Input: dimensioned drawing with shaded views. Units: mm. Origin: part minimum x, y, z. A direction names the side the tool comes from. Round coordinates to 2 decimals unless told otherwise and drop trailing zeros. Loops run counter-clockwise (first coordinate to the right, second up) from the corner with the lowest first, then second, coordinate; pieces in that order, holes last. Notation, with made-up numbers: M -7.75,-24.5 L 19.25,-24.5 A16 ccw 19.25,-15.5 Z; hole C 35,54.5 d7. An arc over 180 degrees is marked long. Write each question's results on one line, items separated by ' | '. Start each with the question number.
1. Section D-D on x = 3. Output: boundary loops of the cut face in (y, z).
2. Draft query along X for the marked faces 1, 2 and 3. Return one class per face: released by +X, released by -X, zero draft, split by the parting line, or undercut.
3. Set-up query: the marked faces 4, 5 and 6. Return all of +Z, -Z, +X, -X, +Y, -Y with unobstructed straight access to the full face (end or side cutting, diameter ignored); none if empty.
4. Section C-C on x = 25. Output: boundary loops of the cut face in (y, z) (1 decimal).
5. Contact query for flat-ended pins moving along their axis: pin 1 Ø1 at (x, z) = (12, 4.5) entering from +Y; pin 2 Ø1.6 at (x, z) = (22.5, 4) entering from +Y (1 decimal); pin 3 Ø1.5 at (y, z) = (15.5, 3.5) entering from -X. Output: stop coordinate, or through.
6. Section A-A on z = 3.35. Output: boundary loops of the cut face in (x, y) (1 decimal).
7. Ray query, line 1 (Y direction, x = 15.75, z = 2.8); line 2 (X direction, y = 14, z = 4.4); line 3 (Z direction, x = 17.5, y = 10.25). Return the intervals inside material, ascending.
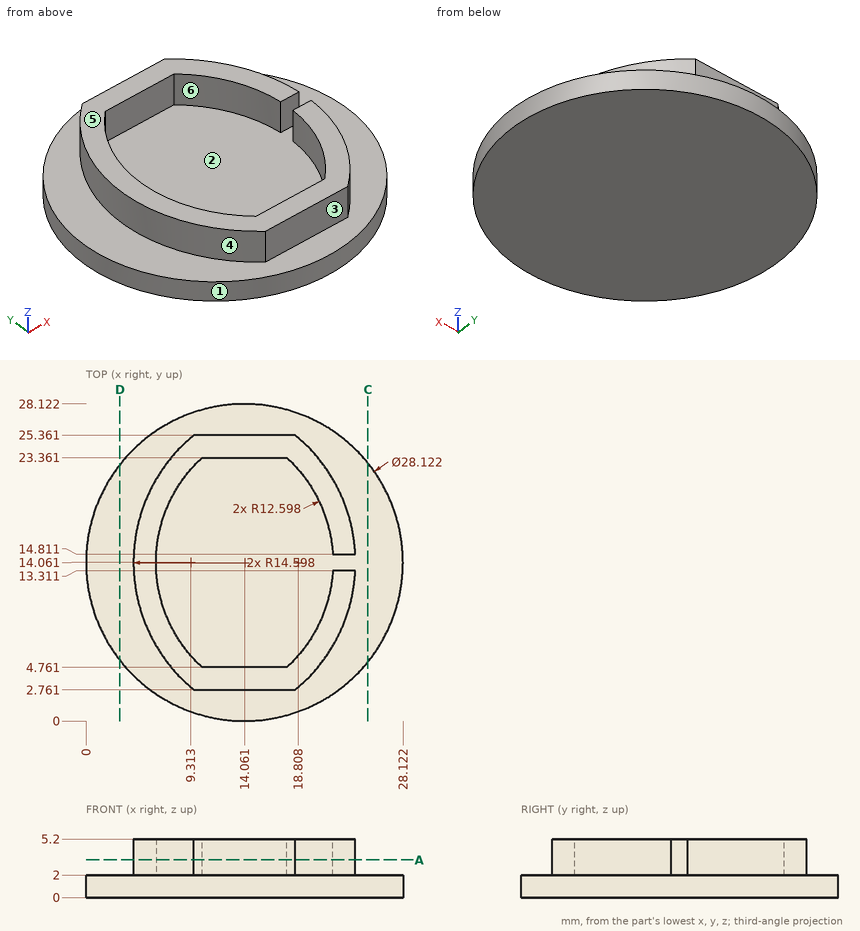
Taken from the geometry:
1) outline: M 5.38,0 L 22.74,0 L 22.74,2 L 5.38,2 Z
2) face 1: split by the parting line | face 2: undercut | face 3: zero draft
3) face 4: +Z, -X | face 5: +Z, +X, -X, +Y, -Y | face 6: +Z
4) outline: M 5.2,0 L 22.9,0 L 22.9,2 L 5.2,2 Z
5) pin 1: y = 25.36 | pin 2: y = 21.8 | pin 3: x = 4.23
6) outline: M 9.6,2.8 L 18.6,2.8 A14.6 ccw 23.9,13.3 L 21.9,13.3 A12.6 cw 17.8,4.8 L 10.3,4.8 A12.6 cw 10.3,23.4 L 17.8,23.4 A12.6 cw 21.9,14.8 L 23.9,14.8 A14.6 ccw 18.6,25.4 L 9.6,25.4 A14.6 ccw Z
7) line 1: 2.76 to 4.76, 23.36 to 25.36 | line 2: 4.21 to 6.21 | line 3: 0 to 2
